Autodesk Inventor part; units mm, degrees
ref_plane "YZ Plane" through (0, 0, 0) normal (1, 0, 0) x (0, 1, 0)
ref_plane "XZ Plane" through (0, 0, 0) normal (0, 1, 0) x (-1, 0, 0)
ref_plane "XY Plane" through (0, 0, 0) normal (0, 0, 1) x (1, 0, 0)
sketch "Sketch1" plane through (0, 0, 0) normal (0, 1, 0) x (-1, 0, 0)
  line L0 (-14.224, 22.225) -> (14.224, 22.225)
  line L1 (14.224, 22.225) -> (14.224, -22.225)
  line L2 (14.224, -22.225) -> (-14.224, -22.225)
  line L3 (-14.224, -22.225) -> (-14.224, 22.225)
  line L4 (-14.224, 22.225) -> (14.224, -22.225) construction
  line L5 (14.224, 22.225) -> (-14.224, -22.225) construction
  point P0 (0, 0)
  dimension "d0" = 28.448
  dimension "d1" = 44.45
extrude "Extrusion1" add sketch "Sketch1" along normal blind 44.45
sketch "Sketch2" plane through (-14.224, 0, 22.225) normal (0, 0, 1) x (1, 0, 0)
  line L0 (12.7, 34.798) -> (53.9197, 34.798)
  line L1 (53.9197, 34.798) -> (53.9197, 9.652)
  line L2 (53.9197, 9.652) -> (12.7, 9.652)
  line L3 (12.7, 9.652) -> (12.7, 34.798)
  line L4 (0, 0) -> (0, 44.45)
  line L5 (0, 44.45) -> (28.448, 44.45)
  line L6 (0, 0) -> (28.448, 0)
  point P0 (14.224, 0)
  dimension "d4" = 12.7
  dimension "d5" = 9.652
  dimension "d6" = 9.652
extrude "Extrusion2" cut sketch "Sketch2" against normal blind 44.45
sketch "Sketch3" plane through (-14.224, 0, -22.225) normal (-1, 0, 0) x (0, 0, 1)
  line L0 (44.45, 22.352) -> (1.7207, 47.0218)
  line L1 (1.7207, 47.0218) -> (53.9201, 57.7184)
  line L2 (53.9201, 57.7184) -> (44.45, 22.352)
  line L3 (0, 0) -> (44.45, 0)
  line L4 (0, 44.45) -> (44.45, 44.45)
  point P0 (22.225, 0)
  dimension "d9" = 22.352
extrude "Extrusion3" cut sketch "Sketch3" against normal through all
properties part number "SLIDE"
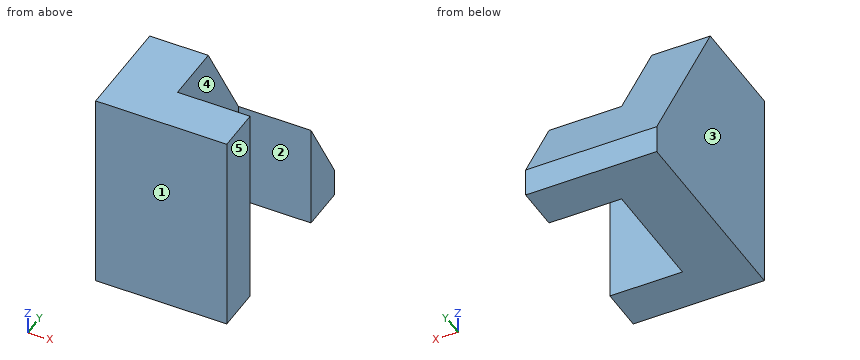
Input: part model. Units: mm. Frame: model coordinates. Face numbers are marked on the shaded views. A direction names the side the tool comes from. Coordinates: 2 decimals unless noted, no trailing zeros. Loops run counter-clockwise (first coordinate to the right, second up) from the corner with the lowest first, then second, coordinate; pieces in that order, holes last. Notation, with made-up numbers: (53, 72.5) - (88, 72.5) arc R23 cw to (88, 103.5) - close; hole circle Ø7 at (88, -36). An arc over 180 degrees is marked (long way). Answer in a Markdown table with one row per item. Add a question column.
Item 1: Mould query, pull axis Y, two halves, no side actions, for the marked faces 1, 2 and 3. Classes: released by +Y, released by -Y, zero draft, split by the parting line, or undercut.
Item 2: Section query B-B on z = -9.5. Return the cut outline in (x, y), then the cut area to 3 significant figures.
Item 3: Section query A-A on x = 2. Return the cut outline in (y, z) (3 decimals), then the cut area to 3 significant figures.
Item 4: Line query: line 1 along Y through (x, z) = (11, -19.5); line 2 along X through (y, z) = (30.5, 7.5); line 3 along Y through (x, z) = (5.75, 15.5). Output: solid intervals per line, ascending. Write a range as [from, to].
Item 5: Section query D-D on x = -8. Return the cut outline in (y, z) (3 decimals).
Item 6: Contact query for flat-ended pins moving along their axis: P1, Ø6, axis at x = -8.5, z = 5, coming from the +Y side; P2, Ø6, axis at x = -1, z = -9.5, coming from the +Y side; P3, Ø12.5, axis at y = 23.5, z = -1.5, coming from the +X side. Output: stop coordinate, or through.
Item 7: Section query C-C on y = 12.5. Return the cut outline in (x, z) (3 decimals), then the cut area to 3 significant figures.
Item 8: Access query for the marked faces 4 and 5. Directions: +Z, -Z, +X, -X, +Y, -Y. A direction counts if a zero-diameter tool reaches every point of the face in a straight line with its end or side. Return the directions, or none.
Recorded:
| question | item | result |
|---|---|---|
| 1 | face 1 | released by -Y |
| 1 | face 2 | undercut |
| 1 | face 3 | zero draft |
| 2 | outline | (-14.22, 0) - (14.22, 0) - (14.22, 9.65) - (-1.52, 9.65) - (-1.52, 34.8) - (14.22, 34.8) - (14.22, 40.67) - (-14.22, 40.67) - close |
| 2 | area | 761 mm^2 |
| 3 | outline | (0, -22.225) - (9.652, -22.225) - (9.652, 22.225) - (0, 22.225) - close; (34.798, -22.225) - (44.45, -22.225) - (44.45, -16.05) - (34.798, 0.668) - close |
| 3 | area | 569 mm^2 |
| 4 | line 1 | [0, 9.65], [34.8, 44.45] |
| 4 | line 2 | [-14.22, -1.52] |
| 4 | line 3 | [0, 9.65] |
| 5 | outline | (0, -22.225) - (44.45, -22.225) - (44.45, -16.05) - (22.352, 22.225) - (0, 22.225) - close |
| 6 | P1 | y = 34.03 |
| 6 | P2 | y = 42.4 |
| 6 | P3 | x = -1.52 |
| 7 | outline | (-14.224, -22.225) - (-1.524, -22.225) - (-1.524, 22.225) - (-14.224, 22.225) - close |
| 7 | area | 565 mm^2 |
| 8 | face 4 | +Z, -Z, +X |
| 8 | face 5 | +Z, -Z, +X, +Y, -Y |
